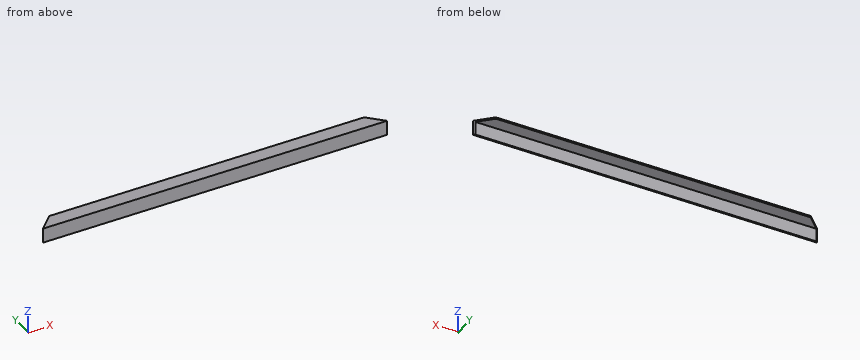
from build123d import *

# Parameters (mm, degrees)
EXTRUDE_1_DEPTH     = 353
CUT_EXTRUDE_1_DEPTH = 16


with BuildPart() as part:
    # Эскиз1 → Бобышка-Вытянуть1 (new body)
    with BuildSketch(Plane(origin=(0, 0, 0), x_dir=(0, 0, -1), z_dir=(1, 0, 0))):
        Polygon((0, 0), (0, 15), (1.5, 15), (1.5, 1.5), (15, 1.5), (15, 0), align=None)
    extrude(amount=EXTRUDE_1_DEPTH)

    # Эскиз2 → Вырез-Вытянуть1 (cut, through all)
    with BuildSketch(Plane.XY):
        Polygon((0, 0), (21.729873861, 21.729873861), (0, 21.729873861), align=None)
    cut_extrude_1 = extrude(amount=-CUT_EXTRUDE_1_DEPTH, mode=Mode.SUBTRACT)

    # Зеркальное отражение1: Вырез-Вытянуть1 across plane
    add(cut_extrude_1.mirror(Plane.ZY.offset(-176.5)), mode=Mode.SUBTRACT)


solid = part.part
Geometry: final body of the model. Coordinates: model frame, mm. Coordinates: 2 decimals unless noted, no trailing zeros. Loops run counter-clockwise (first coordinate to the right, second up) from the corner with the lowest first, then second, coordinate; pieces in that order, holes last. Notation, with made-up numbers: (-14.5, -8.5) - (-8.5, -8.5) arc R17 ccw to (-8.5, -1.5) - close; hole circle Ø4 at (23, -20.5). An arc over 180 degrees is marked (long way). Put each result on its own line as item: value. Start each with the question number.
Q1. Line query: line 1 (Y direction, x = 330.5, z = -9.75); line 2 (Z direction, x = 233.5, y = 7); line 3 (X direction, y = 0.75, z = -1.75). Output: solid intervals per line, ascending.
Q2. Cut plane B-B, the plane y = 6.5. Return loops of the section in (x, z).
Q3. Pin query (flat end, axial travel): pin 1 Ø4 at (x, y) = (43, 11) entering from -Z; pin 2 Ø3 at (y, z) = (2.5, -6) entering from +X; pin 3 Ø4 at (x, z) = (154, -9) entering from +Y. Return the tip coordinate at first contact, or that it passes through.
Q4. Cut plane A-A, the plane x = 143.5. Return loops of the section in (y, z), and give its area (4 significant figures).
Q5. Cut plane C-C, the plane z = -6.75. Return loops of the section in (x, y).
Filled sheet:
1. line 1: 0 to 1.5
1. line 2: -1.5 to 0
1. line 3: 0.75 to 352.25
2. outline: (6.5, -1.5) - (346.5, -1.5) - (346.5, 0) - (6.5, 0) - close
3. pin 1: z = -1.5
3. pin 2: x = 352
3. pin 3: y = 1.5
4. outline: (0, -15) - (1.5, -15) - (1.5, -1.5) - (15, -1.5) - (15, 0) - (0, 0) - close
4. area: 42.75 mm²
5. outline: (0, 0) - (353, 0) - (351.5, 1.5) - (1.5, 1.5) - close
